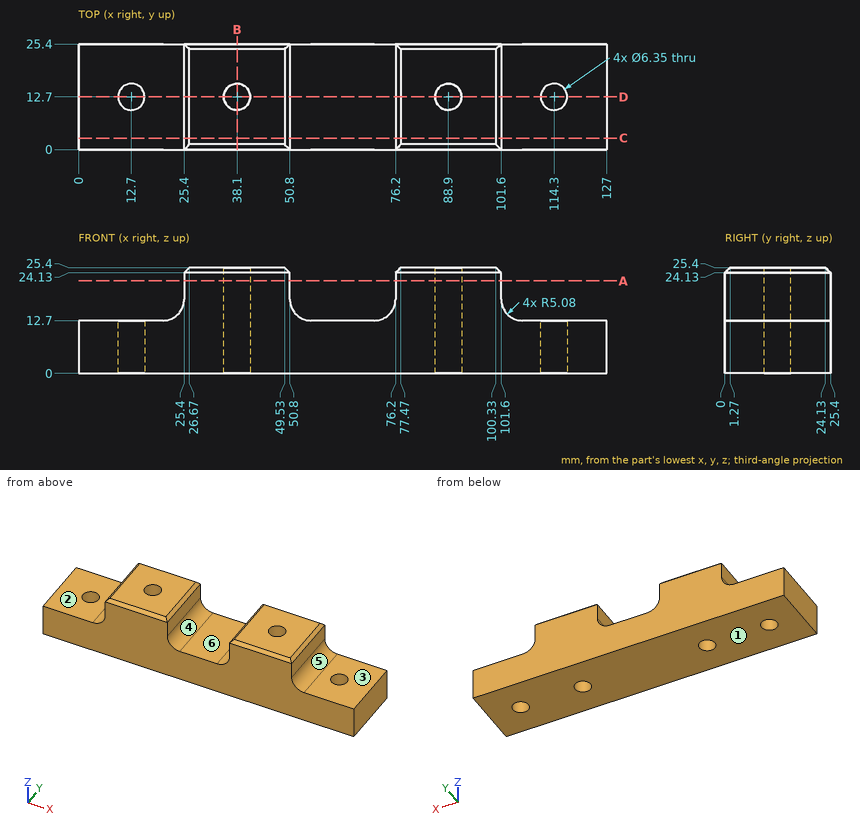
The figure shows three views and two pictorial views of one solid part (mm, origin at its lowest corner). Answer the questions. A direction names the side the tool comes from. Give positions to 0.01 mm unless a question says otherwise; leave off trailing zeros. Loops run counter-clockwise (first coordinate to the right, second up) from the corner with the lowest first, then second, coordinate; pieces in that order, holes last. Notation, with made-up numbers: (74.5, 61) -> (94.5, 61) arc R33 ccw to (94.5, 97) -> close; hole circle Ø5 at (-10.5, 2). An arc over 180 degrees is marked (long way). Put each result on its own line as item: value. Start each with the question number.
Item 1: The mould has two halves that part along X. Classify the marked faces 3, 4, 5 and 6: released by +X, released by -X, zero draft, split by the parting line, or undercut.
Item 2: The part is cut by section C-C (y = 2.75). Give the vertices of the cut face in (x, z), then the cut area to 3 significant figures.
Item 3: The part is cut by section B-B (x = 38.1). Give the vertices of the cut face in (y, z) (3 decimals), then the cut area to 3 significant figures.
Item 4: Each of these flat-tipped pins is pushed along its axis until it touches: P1, Ø10, axis at x = 8.5, y = 12.5, coming from the +Z side; P2, Ø1.9, axis at y = 9, z = 20, coming from the +X side; P3, Ø5, axis at y = 10.5, z = 22.5, coming from the -X side. Where does it stop, or does it pass through?
Item 5: Which of the six approach directions +Z, -Z, +X, -X, +Y, -Y give full straight-line access (tool end or side, diameter ignored) to the marked faces 1 and 2?
Item 6: The part is cut by section A-A (z = 22.25). Give the vertices of the cut face in (x, y) (3 decimals).
Item 7: The part is cut by section D-D (y = 12.7). State how many separate pieces and enclosed holes the cut face has, then the cut area to 3 significant figures.
Item 8: Find the intervals of material crossed by L1, parallel to Y at x = 114.3, z = 6.25 (3 decimals); L2, parallel to X at y = 23.75, z = 17.75; L3, parallel to Z at x = 59, y = 11, in increasing order. Write a range as [from, to].
Answers below:
1. face 3: zero draft
1. face 4: undercut
1. face 5: released by +X
1. face 6: undercut
2. outline: (0, 0) -> (127, 0) -> (127, 12.7) -> (106.68, 12.7) arc R5.08 cw to (101.6, 17.78) -> (101.6, 24.13) -> (100.33, 25.4) -> (77.47, 25.4) -> (76.2, 24.13) -> (76.2, 17.78) arc R5.08 cw to (71.12, 12.7) -> (55.88, 12.7) arc R5.08 cw to (50.8, 17.78) -> (50.8, 24.13) -> (49.53, 25.4) -> (26.67, 25.4) -> (25.4, 24.13) -> (25.4, 17.78) arc R5.08 cw to (20.32, 12.7) -> (0, 12.7) -> close
2. area: 2,280 mm2
3. outline: (0, 0) -> (9.525, 0) -> (9.525, 25.4) -> (1.27, 25.4) -> (0, 24.13) -> close; (15.875, 0) -> (25.4, 0) -> (25.4, 24.13) -> (24.13, 25.4) -> (15.875, 25.4) -> close
3. area: 482 mm2
4. P1: z = 12.7
4. P2: x = 101.6
4. P3: x = 25.4
5. face 1: -Z, +X, -X, +Y, -Y
5. face 2: +Z, -X, +Y, -Y
6. outline: (25.4, 0) -> (50.8, 0) -> (50.8, 25.4) -> (25.4, 25.4) -> close; (76.2, 0) -> (101.6, 0) -> (101.6, 25.4) -> (76.2, 25.4) -> close; hole circle Ø6.35 at (38.1, 12.7); hole circle Ø6.35 at (88.9, 12.7)
7. separate pieces: 5
7. enclosed holes: 0
7. area: 1,790 mm2
8. L1: [0, 9.525], [15.875, 25.4]
8. L2: [25.4, 50.8], [76.2, 101.6]
8. L3: [0, 12.7]
